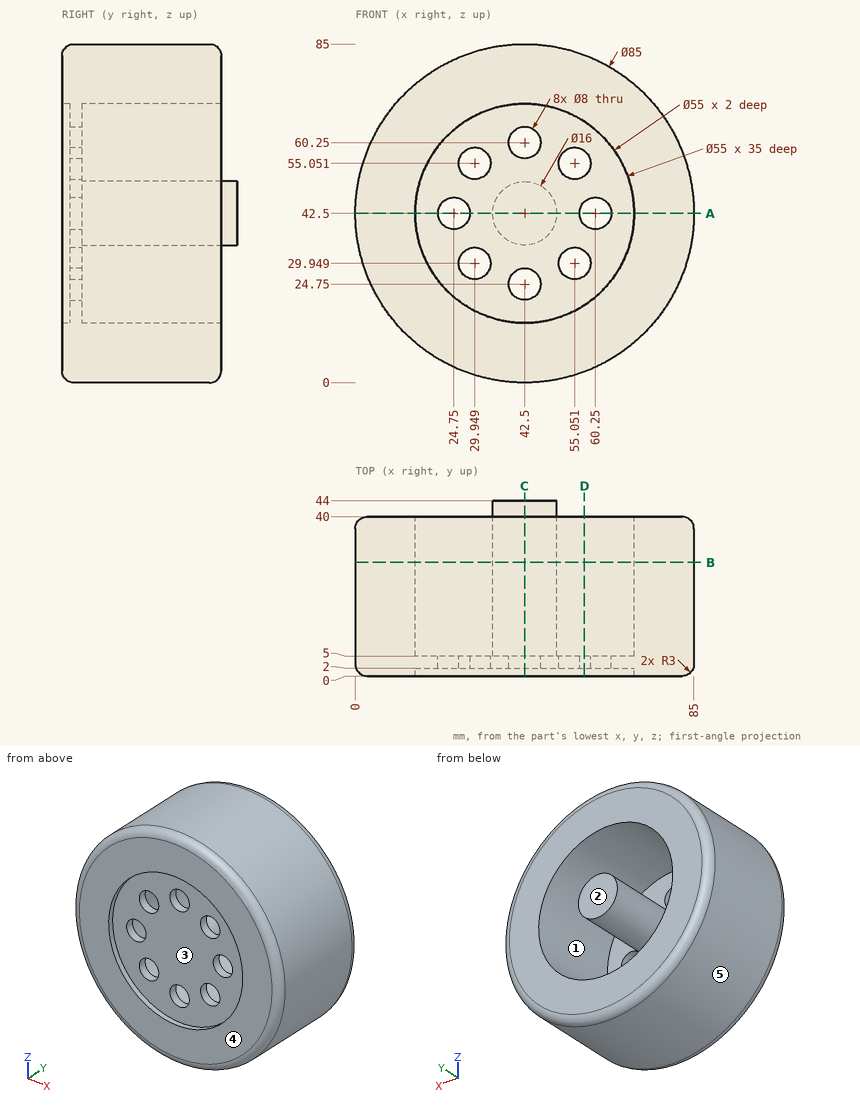
Drawing for the job (mm, zero at the part's lowest x, y, z). A direction names the side the tool comes from. Give positions to 0.01 mm unless a question says otherwise; leave off trailing zeros. Loops run counter-clockwise (first coordinate to the right, second up) from the corner with the lowest first, then second, coordinate; pieces in that order, holes last. Notation, with made-up numbers: M -8.75,-22.75 L 17.25,-22.75 A16 ccw 17.25,-12.75 Z; hole C 43,-6.5 d2. An arc over 180 degrees is marked long. One line per question, with ' | ' between items. Start each with the question number.
1. Two-plate mould, pull along X, no slides. Class the marked faces 3, 4 and 5: pulls with the +X half, pulls with the -X half, needs draft (parallel to the pull), parting line crosses it, or undercut.
2. Saw through at A-A on z = 42.5. Give the cut face in (x, y).
3. 3-axis set-ups, long thin cutter, end or side, ignore diameter. For the marked faces 1 and 2: which of +Z, -Z, +X, -X, +Y, -Y reach the whole face in a straight line?
4. Saw through at B-B on y = 28.5. Give the cut face in (x, z), plus the area to 3 significant figures.
5. Probe L1, parallel to X at y = 22, z = 42.5; L2, parallel to Z at x = 43.5, y = 10.5; L3, parallel to X at y = 14, z = 35.5 (1 decimal). List the from-to ranges inside material, lowest first. Write a range as from..to.
6. Saw through at D-D on x = 57.5. State how many separate pieces and enclosed holes the cut face has, plus the area to 3 significant figures.
7. Flat gauge pins, fed straight in: pin 1 (10 mm diameter, centred on x = 30, y = 7, fed in from -Z); pin 2 (10 mm diameter, centred on x = 27.5, z = 70.5, fed in from +Y); pin 3 (13 mm diameter, centred on x = 60.25, z = 42.5, fed in from -Y). Where does each tip first touch, or does it go through?
8. Saw through at C-C on x = 42.5. Give the cut face in (y, z).
Result sheet:
1) face 3: undercut | face 4: needs draft | face 5: parting line crosses it
2) outline: M 0,3 A3 ccw 3,0 L 15,0 L 15,2 L 20.75,2 L 20.75,5 L 15,5 L 15,40 L 3,40 A3 ccw 0,37 Z; M 28.75,2 L 56.25,2 L 56.25,5 L 50.5,5 L 50.5,44 L 34.5,44 L 34.5,5 L 28.75,5 Z; M 64.25,2 L 70,2 L 70,0 L 82,0 A3 ccw 85,3 L 85,37 A3 ccw 82,40 L 70,40 L 70,5 L 64.25,5 Z
3) face 1: +Y | face 2: +Z, -Z, +X, -X, +Y
4) outline: C 42.5,42.5 d85; C 42.5,42.5 d16; hole C 42.5,42.5 d55 | area: 3,500 mm^2
5) L1: x = 0..15, 34.5..50.5, 70..85 | L2: z = 0.01..15.02, 34.56..50.44, 69.98..84.99 | L3: x = 0.6..15.9, 38.6..46.4, 69.1..84.4
6) separate pieces: 4 | enclosed holes: 0 | area: 1,410 mm^2
7) pin 1: stops at z = 0.67 | pin 2: stops at y = 40 | pin 3: stops at y = 2
8) outline: M 0,3 A3 ccw 3,0 L 37,0 A3 ccw 40,3 L 40,15 L 5,15 L 5,20.75 L 2,20.75 L 2,15 L 0,15 Z; M 0,70 L 2,70 L 2,64.25 L 5,64.25 L 5,70 L 40,70 L 40,82 A3 ccw 37,85 L 3,85 A3 ccw 0,82 Z; M 2,28.75 L 5,28.75 L 5,34.5 L 44,34.5 L 44,50.5 L 5,50.5 L 5,56.25 L 2,56.25 Z
